Geometry: see drawing. Coordinates: mm, zero at the bounding-box minimum. Round coordinates to 2 decimals unless told otherwise and drop trailing zeros. Write each loop counter-clockwise with the first axis right and the second up, starting at its lowest first coordinate (ties: lowest second). Pieces come first, ordered by that corner, then holes. Notation, with made-up numbers: (25, 56.25) -> (53, 56.25) arc R24 ccw to (53, 85.25) -> close; hole circle Ø5 at (0.5, 65). An arc over 180 degrees is marked (long way). Write item = value, one per line.
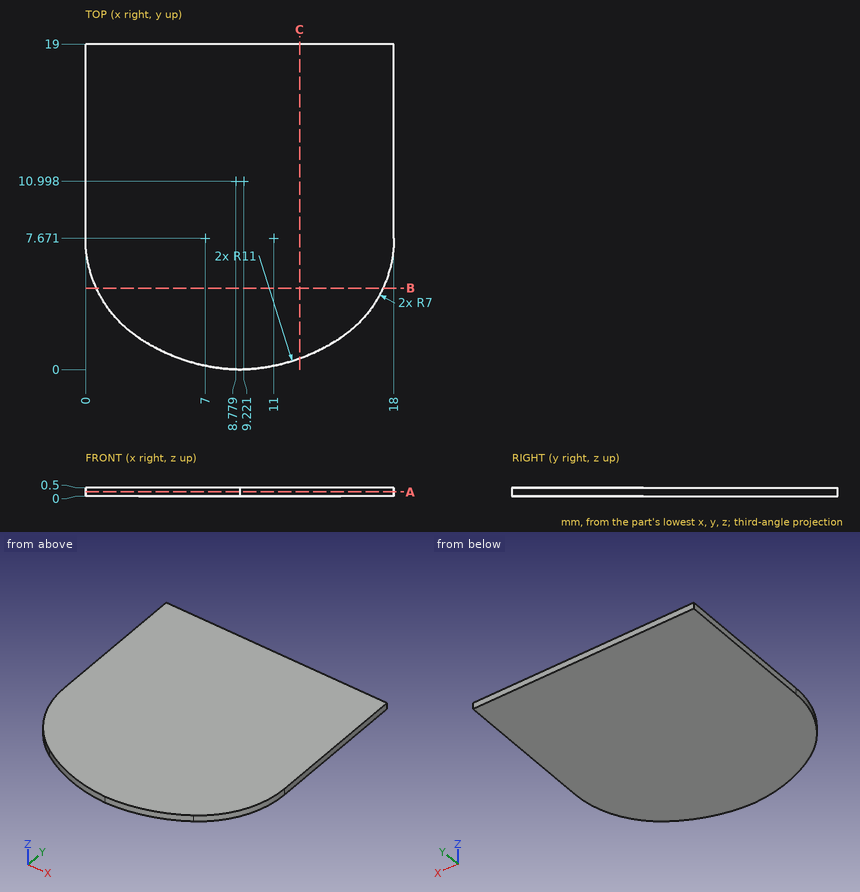
1) Cut plane B-B (y = 4.75). Return the cut outline in (x, z).
Solutions:
outline = (0.64, 0) -> (17.36, 0) -> (17.36, 0.5) -> (0.64, 0.5) -> close
2) Cut plane C-C (x = 12.5). Return the cut outline in (y, z).
Solutions:
outline = (0.65, 0) -> (19, 0) -> (19, 0.5) -> (0.65, 0.5) -> close
3) Cut plane A-A (z = 0.25). Return the cut outline in (x, y), and give its area (4 significant figures).
Solutions:
outline = (0, 7.67) arc R7 ccw to (3.11, 1.85) arc R11 ccw to (9, 0) arc R11 ccw to (14.89, 1.85) arc R7 ccw to (18, 7.67) -> (18, 19) -> (0, 19) -> close
area = 312.5 mm^2
4) Line query: L1, parallel to X at y = 6.5, z = 0.1; L2, parallel to Y at x = 10, z = 0.4; L3, parallel to Y at x = 2.5, z = 0.1. Output: solid intervals per line, ascending. Write a range as from..to.
Solutions:
L1 = 0.1..17.9
L2 = 0.07..19
L3 = 2.31..19
